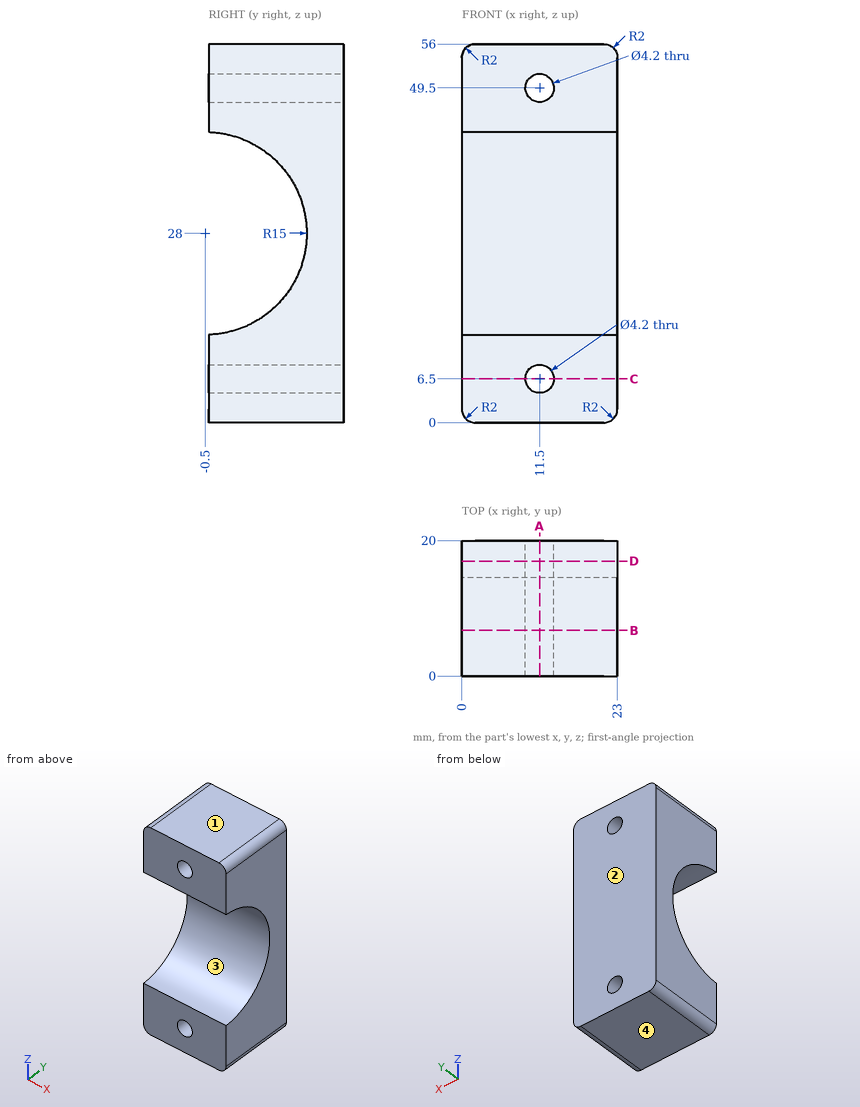
Verification items for this drawing (mm, ordinates from the low corner). Round coordinates to 2 decimals unless told otherwise and drop trailing zeros. Loops run counter-clockwise (first coordinate to the right, second up) from the corner with the lowest first, then second, coordinate; pieces in that order, holes last. Notation, with made-up numbers: (13.5, 71) - (18.5, 71) arc R20 cw to (18.5, 82) - close; hole circle Ø8 at (-21, -34). An arc over 180 degrees is marked (long way). Write item = value, one per line.
Q1. Sectioned sample at D-D on y = 17. Record the boundary of the cut face in (x, z).
Here are the results:
outline = (0, 2) arc R2 ccw to (2, 0) - (21, 0) arc R2 ccw to (23, 2) - (23, 54) arc R2 ccw to (21, 56) - (2, 56) arc R2 ccw to (0, 54) - close; hole circle Ø4.2 at (11.5, 6.5); hole circle Ø4.2 at (11.5, 49.5)
Q2. Mould release check, pull along Z, two halves, no side actions. Record for the marked faces 1, 2, 3 and 4: +Z half, -Z half, draft (parallel to the pull), parting line (faces both ways), or undercut.
Here are the results:
face_1 = +Z half
face_2 = draft
face_3 = undercut
face_4 = -Z half
Q3. Sectioned sample at B-B on y = 6.75. Record the boundary of the cut face in (x, z), plus the area to 3 significant figures.
Here are the results:
outline = (0, 2) arc R2 ccw to (2, 0) - (21, 0) arc R2 ccw to (23, 2) - (23, 14.87) - (0, 14.87) - close; (0, 41.13) - (23, 41.13) - (23, 54) arc R2 ccw to (21, 56) - (2, 56) arc R2 ccw to (0, 54) - close; hole circle Ø4.2 at (11.5, 6.5); hole circle Ø4.2 at (11.5, 49.5)
area = 653 mm^2
Q4. Material ranges on L1, parallel to X at y = 15.75, z = 6.5; L2, parallel to Z at x = 11.5, y = 10.75; L3, parallel to Z at x = 11.5, y = 7, recorded low to high.
Here are the results:
L1 = 0 to 9.4, 13.6 to 23
L2 = 0 to 4.4, 8.6 to 18.08, 37.92 to 47.4, 51.6 to 56
L3 = 0 to 4.4, 8.6 to 15.01, 40.99 to 47.4, 51.6 to 56
Q5. Sectioned sample at C-C on z = 6.5. Record the boundary of the cut face in (x, y), plus the area to 3 significant figures.
Here are the results:
outline = (0, 0) - (9.4, 0) - (9.4, 20) - (0, 20) - close; (13.6, 0) - (23, 0) - (23, 20) - (13.6, 20) - close
area = 376 mm^2
Q6. Depth check by flat-ended pin: pin 1 (4 mm diameter, centred on x = 11.5, z = 6.5, fed in from +Y). Enter the tip coordinate at first touch or a pass-through.
Here are the results:
pin_1 = through
Q7. Sectioned sample at A-A on x = 11.5. Record the boundary of the cut face in (y, z).
Here are the results:
outline = (0, 0) - (20, 0) - (20, 4.4) - (0, 4.4) - close; (0, 8.6) - (20, 8.6) - (20, 47.4) - (0, 47.4) - (0, 42.99) arc R15 cw to (0, 13.01) - close; (0, 51.6) - (20, 51.6) - (20, 56) - (0, 56) - close
